```python
from build123d import *

# Parameters (mm, degrees)
F1_DEPTH = 45
F3_DEPTH = 30
F4_DEPTH = 3
F6_DEPTH = 3
F7_R     = 1
F8_R     = 0.2


with BuildPart() as f1:
    # F0 (on Top) → F1 (new body)
    with BuildSketch(Plane.XY):
        with BuildLine():
            Line((-22.0269914716, 9.8525723957), (8.9730085284, 9.8525723957))
            Line((8.9730085284, 9.8525723957), (8.9730085284, -40.1474276043))
            Line((8.9730085284, -40.1474276043), (11.9730085284, -40.1474276043))
            Line((11.9730085284, -40.1474276043), (11.9730085284, 13.0525723957))
            Line((11.9730085284, 13.0525723957), (-25.0269914716, 13.0525723957))
            Line((-25.0269914716, 13.0525723957), (-25.0269914716, -7.4474276043))
            ThreePointArc((-25.0269914716, -7.4474276043), (-21.791751143, -5.2297159987), (-19.0269914716, -2.4474276043))
            Line((-19.0269914716, -2.4474276043), (-22.0269914716, -2.4474276043))
            Line((-22.0269914716, -2.4474276043), (-22.0269914716, 9.8525723957))
        make_face()
    extrude(amount=F1_DEPTH)

    # F2 (on face) → F3 (join)
    with BuildSketch(Plane.YZ.offset(11.9730085284)):
        with BuildLine():
            Line((-40.1474276043, 0), (-36.1474276043, 0))
            ThreePointArc((-36.1474276043, 0), (-32.1289821926, 22.5), (-36.1474276043, 45))
            Line((-36.1474276043, 45), (-40.1474276043, 45))
            ThreePointArc((-40.1474276043, 45), (-36.1289821926, 22.5), (-40.1474276043, 0))
        make_face()
    extrude(amount=F3_DEPTH)

    # F4 (cut): a face of the model
    f4_faces = [f1.faces().sort_by_distance(p)[0] for p in [
        (11.9730085284, -38.5357130978, 22.5),
    ]]
    extrude(f4_faces, amount=-F4_DEPTH, mode=Mode.SUBTRACT)

    # F5 (on face) → F6 (join)
    with BuildSketch(Plane.YZ.offset(41.9730085284)):
        with BuildLine():
            ThreePointArc((-40.1474276043, 45), (-36.1289821926, 22.5), (-40.1474276043, 0))
            Line((-40.1474276043, 0), (-8.1474276043, 0))
            ThreePointArc((-8.1474276043, 0), (-4.1289821926, 22.5), (-8.1474276043, 45))
            Line((-8.1474276043, 45), (-40.1474276043, 45))
        make_face()
    extrude(amount=F6_DEPTH)

    # F7
    f7_edges = [f1.edges().sort_by_distance(p)[0] for p in [
        (11.973009, 13.052572, 22.5),
        (-25.026991, 13.052572, 22.5),
        (-22.026991, 9.852572, 22.5),
        (8.973009, 9.852572, 22.5),
        (8.973009, -36.128982, 22.5),
        (44.973009, -36.128982, 22.5),
        (44.973009, -4.128982, 22.5),
        (41.973009, -4.128982, 22.5),
        (41.973009, -32.128982, 22.5),
        (11.973009, -32.128982, 22.5),
    ]]
    fillet(f7_edges, radius=F7_R)

    # F8
    f8_edges = [f1.edges().sort_by_distance(p)[0] for p in [
        (-19.026991, -2.447428, 22.5),
        (-25.026991, -7.447428, 22.5),
    ]]
    fillet(f8_edges, radius=F8_R)


solid = f1.part
```
Part model, mm, in its own coordinate system. A direction names the side the tool comes from. Round coordinates to 2 decimals unless told otherwise and drop trailing zeros. Order: outer loops, then holes, each group sorted by start corner. A loop starts at its lowest first (then second) coordinate and runs counter-clockwise, first axis right, second up. Notation, with made-up numbers: M -39,23.5 L 3,23.5 A33 cw 3,60.5 Z; hole C 69,56.25 d8. An arc over 180 degrees is marked long. Put each result on its own line as item: value. Start each with the question number.
1. Drill centre lines: probe 1 along X at (y, z) = (-30, 27.5); probe 2 along X at (y, z) = (9, 40); probe 3 along Y at (x, z) = (0, 28). Where is each one in solid material? Low to high. Write a range as [from, to].
2. Slice it at D-D on x = 2. List the corners of the cut face in (y, z).
3. Slice it at A-A on y = -12.5. List the corners of the cut face in (x, z), then the cut area to 3 significant figures.
4. Tool access for faces 1 (the face through (-6, 13.053, 22)), 2 (the face through (8.973, -15, 22)), 3 (the face through (10, -14, 0)), 4 (the face through (26.78, -32.13, 22.18)), 5 (the face through (-22.027, 3, 22)): list every direction of +Z, -Z, +X, -X, +Y, -Y with a clear straight run to the whole face (end or side of a thin tool).
5. Slice it at C-C on x = 24.5. List the corners of the cut face in (y, z), then the cut area to 3 significant figures.
6. Two-plate mould, pull along X, no slides. Class faces 6 (the face through (44.973, -22, 23)), 7 (the face through (-21.863, -5.289, 22.185)), 8 (the face through (43.47, -4.13, 22.18)): +X half, -X half, draft (parallel to the pull), parting line (faces both ways), or undercut.
7. Drop flat-ended pins along their axis: pin 1 (12 mm diameter, centred on x = 20, z = 34, fed in from +Y); pin 2 (5.5 mm diameter, centred on y = 1, z = 18, fed in from +X); pin 3 (2 mm diameter, centred on x = 37.5, z = 21.5, fed in from +Y); pin 4 (8 mm diameter, centred on x = 11.5, z = 23, fed in from +Y). Give the stop position or say it passes through.
8. Slice it at B-B on z = 22.5. List the corners of the cut face in (x, y), then the cut area to 3 significant figures.
Findings:
1. probe 1: [8.97, 11.97], [41.97, 44.97]
1. probe 2: [-25.03, -22.02], [8.96, 11.97]
1. probe 3: [9.85, 13.05]
2. outline: M 9.85,0 L 13.05,0 L 13.05,45 L 9.85,45 Z
3. outline: M 8.97,0 L 11.97,0 L 11.97,45 L 8.97,45 Z; M 41.97,0 L 44.97,0 L 44.97,45 L 41.97,45 Z
3. area: 270 mm2
4. face 1: +Z, -Z, +X, -X, +Y
4. face 2: +Z, -Z, -Y
4. face 3: -Z, +X, -X, +Y, -Y
4. face 4: +Y
4. face 5: +Z, -Z
5. outline: M -40.15,0 L -36.15,0 A65 ccw -36.15,45 L -40.15,45 A65 cw Z
5. area: 180 mm2
6. face 6: +X half
6. face 7: undercut
6. face 8: draft
7. pin 1: y = -32.36
7. pin 2: x = 11.97
7. pin 3: y = -32.13
7. pin 4: y = 13.05
8. outline: M -25.03,-7.1 A0.2 ccw -24.73,-7.28 A20.93 ccw -19.3,-2.78 A0.2 ccw -19.46,-2.45 L -22.03,-2.45 L -22.03,8.85 A1 cw -21.03,9.85 L 7.97,9.85 A1 cw 8.97,8.85 L 8.97,-35.13 A1 ccw 9.97,-36.13 L 43.97,-36.13 A1 ccw 44.97,-35.13 L 44.97,-5.13 A1 ccw 43.97,-4.13 L 42.97,-4.13 A1 ccw 41.97,-5.13 L 41.97,-31.13 A1 cw 40.97,-32.13 L 12.97,-32.13 A1 cw 11.97,-31.13 L 11.97,12.05 A1 ccw 10.97,13.05 L -24.03,13.05 A1 ccw -25.03,12.05 Z
8. area: 526 mm2
